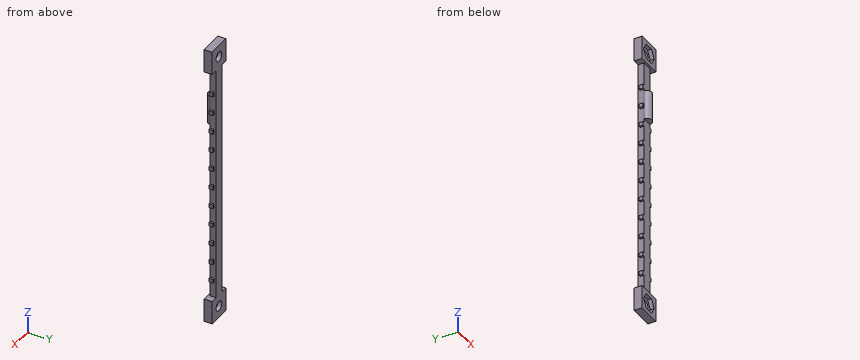
```python
from build123d import *

# Parameters (mm, degrees)
BOSS_EXTRUDE1_DEPTH = 2
BOSS_EXTRUDE2_DEPTH = 1
SKETCH3_W           = 12
SKETCH3_H           = 12
BOSS_EXTRUDE3_DEPTH = 1
CUT_EXTRUDE1_DEPTH  = 2
SKETCH5_R           = 2.5
CUT_EXTRUDE2_DEPTH  = 5
SKETCH6_W           = 3
SKETCH6_H           = 15
BOSS_EXTRUDE4_DEPTH = 5
CUT_EXTRUDE3_DEPTH  = 30
SKETCH9_W           = 3
SKETCH9_H           = 7
CUT_EXTRUDE5_DEPTH  = 20
SKETCH10_W          = 5
SKETCH10_H          = 15
BOSS_EXTRUDE5_DEPTH = 3
CUT_EXTRUDE7_DEPTH  = 20


with BuildPart() as part:
    # Sketch1 → Boss-Extrude1 (new body)
    with BuildSketch(Plane(origin=(0, 0, 0), x_dir=(1, 0, 0), z_dir=(0, 1, 0))):
        Polygon((7.22672382, 6.096), (7.22672382, 18.096), (6.22672382, 18.096), (6.22672382, 20.096), (7.22672382, 20.096), (7.22672382, 28.096), (6.22672382, 28.096), (6.22672382, 30.096), (7.22672382, 30.096), (7.22672382, 38.096), (6.22672382, 38.096), (6.22672382, 40.096), (7.22672382, 40.096), (7.22672382, 48.096), (6.22672382, 48.096), (6.22672382, 50.096), (7.22672382, 50.096), (7.22672382, 58.096), (6.22672382, 58.096), (6.22672382, 60.096), (7.22672382, 60.096), (7.22672382, 68.096), (6.22672382, 68.096), (6.22672382, 70.096), (7.22672382, 70.096), (7.22672382, 78.096), (6.22672382, 78.096), (6.22672382, 80.096), (7.22672382, 80.096), (7.22672382, 88.096), (6.22672382, 88.096), (6.22672382, 90.096), (7.22672382, 90.096), (7.22672382, 98.096), (6.22672382, 98.096), (6.22672382, 100.096), (7.22672382, 100.096), (7.22672382, 108.096), (6.22672382, 108.096), (6.22672382, 110.096), (7.22672382, 110.096), (7.22672382, 118.096), (6.22672382, 118.096), (6.22672382, 120.096), (7.22672382, 120.096), (7.22672382, 128.096), (3.72672382, 128.096), (3.72672382, 140.096), (15.72672382, 140.096), (15.72672382, 128.096), (12.22672382, 128.096), (12.22672382, 120.096), (13.22672382, 120.096), (13.22672382, 118.096), (12.22672382, 118.096), (12.22672382, 110.096), (13.226723821, 110.096), (13.226723821, 108.096), (12.22672382, 108.096), (12.22672382, 100.096), (13.226723821, 100.096), (13.226723821, 98.096), (12.22672382, 98.096), (12.22672382, 90.096), (13.226723821, 90.096), (13.226723821, 88.096), (12.22672382, 88.096), (12.22672382, 80.096), (13.226723821, 80.096), (13.226723821, 78.096), (12.22672382, 78.096), (12.22672382, 70.096), (13.226723821, 70.096), (13.226723821, 68.096), (12.22672382, 68.096), (12.22672382, 60.096), (13.226723821, 60.096), (13.226723821, 58.096), (12.22672382, 58.096), (12.22672382, 50.096), (13.226723821, 50.096), (13.226723821, 48.096), (12.22672382, 48.096), (12.22672382, 40.096), (13.226723821, 40.096), (13.226723821, 38.096), (12.22672382, 38.096), (12.22672382, 30.096), (13.226723821, 30.096), (13.226723821, 28.096), (12.22672382, 28.096), (12.22672382, 20.096), (13.226723821, 20.096), (13.226723821, 18.096), (12.22672382, 18.096), (12.22672382, 6.096), (15.72672382, 6.096), (15.72672382, -5.904), (3.72672382, -5.904), (3.72672382, 6.096), align=None)
    extrude(amount=BOSS_EXTRUDE1_DEPTH)

    # Sketch2 → Boss-Extrude2 (add)
    with BuildSketch(Plane(origin=(0, 2, 0), x_dir=(1, 0, 0), z_dir=(0, 1, 0))):
        Polygon((3.72672382, 140.096), (15.72672382, 140.096), (15.72672382, 128.096), (12.22672382, 128.096), (12.22672382, 6.096), (15.72672382, 6.096), (15.72672382, -5.904), (3.72672382, -5.904), (3.72672382, 6.096), (7.22672382, 6.096), (7.22672382, 128.096), (3.72672382, 128.096), align=None)
    extrude(amount=BOSS_EXTRUDE2_DEPTH)

    # Sketch3 → Boss-Extrude3 (add)
    with BuildSketch(Plane(origin=(0, 0, 0), x_dir=(-1, 0, 0), z_dir=(0, -1, 0))):
        with Locations((-9.72672382, 134.096)):
            Rectangle(SKETCH3_W, SKETCH3_H)
        with Locations((-9.72672382, 0.096)):
            Rectangle(SKETCH3_W, SKETCH3_H)
    extrude(amount=BOSS_EXTRUDE3_DEPTH)

    # Sketch4 → Cut-Extrude1 (cut)
    with BuildSketch(Plane(origin=(0, -1, 0), x_dir=(-1, 0, 0), z_dir=(0, -1, 0))):
        Polygon((-7.365059478, 138.096), (-11.983861632, 138.096), (-14.293262708, 134.096), (-11.983861632, 130.096), (-7.365059478, 130.096), (-5.055658401, 134.096), align=None)
        Polygon((-7.417322744, 4.096), (-12.036124897, 4.096), (-14.345525974, 0.096), (-12.036124897, -3.904), (-7.417322744, -3.904), (-5.107921667, 0.096), align=None)
    extrude(amount=-CUT_EXTRUDE1_DEPTH, mode=Mode.SUBTRACT)

    # Sketch5 → Cut-Extrude2 (cut)
    with BuildSketch(Plane(origin=(0, 1, 0), x_dir=(-1, 0, 0), z_dir=(0, -1, 0))):
        with Locations(Location((-9.72672382, 0.096, 0), (0, 0, 90))):
            Circle(SKETCH5_R)
        with Locations(Location((-9.72672382, 134.096, 0), (0, 0, 90))):
            Circle(SKETCH5_R)
    extrude(amount=-CUT_EXTRUDE2_DEPTH, mode=Mode.SUBTRACT)

    # Sketch6 → Boss-Extrude4 (add)
    with BuildSketch(Plane(origin=(0, 0, 0), x_dir=(-1, 0, 0), z_dir=(0, -1, 0))):
        with Locations((-9.72672382, 28.596)):
            Rectangle(SKETCH6_W, SKETCH6_H)
    extrude(amount=BOSS_EXTRUDE4_DEPTH)

    # Sketch7 → Cut-Extrude3 (cut)
    with BuildSketch(Plane(origin=(0, 0, -36.096), x_dir=(-1, 0, 0), z_dir=(0, 0, -1))):
        with BuildLine():
            Line((-9.72672381, -5), (-8.22672382, -5))
            Line((-8.22672382, -5), (-8.22672382, -1))
            add(Edge.make_bspline(
                [(-9.72672382, -5), (-8.22672382, -5), (-8.22672382, -1)],
                knots=[6.283185307, 6.283185307, 6.283185307, 7.853981634, 7.853981634, 7.853981634], degree=2, weights=[1, 0.707106781, 1]))
        make_face()
        with BuildLine():
            Line((-11.22672382, -5), (-9.72672381, -5))
            add(Edge.make_bspline(
                [(-11.22672382, -1), (-11.22672382, -5), (-9.72672382, -5)],
                knots=[4.71238898, 4.71238898, 4.71238898, 6.283185307, 6.283185307, 6.283185307], degree=2, weights=[1, 0.707106781, 1]))
            Line((-11.22672382, -1), (-11.22672382, -5))
        make_face()
    extrude(amount=-CUT_EXTRUDE3_DEPTH, mode=Mode.SUBTRACT)

    # Sketch9 → Cut-Extrude5 (cut)
    with BuildSketch(Plane.XY.offset(-21.096)):
        with Locations((9.72672382, -3.5)):
            Rectangle(SKETCH9_W, SKETCH9_H)
    extrude(amount=-CUT_EXTRUDE5_DEPTH, mode=Mode.SUBTRACT)

    # Sketch10 → Boss-Extrude5 (add)
    with BuildSketch(Plane(origin=(0, 0, 0), x_dir=(-1, 0, 0), z_dir=(0, -1, 0))):
        with Locations((-9.72672382, 28.596)):
            Rectangle(SKETCH10_W, SKETCH10_H)
    extrude(amount=BOSS_EXTRUDE5_DEPTH)

    # Sketch11 → Cut-Extrude7 (cut)
    with BuildSketch(Plane(origin=(0, 0, -36.096), x_dir=(-1, 0, 0), z_dir=(0, 0, -1))):
        with BuildLine():
            Line((-7.22672382, -3), (-7.22672382, 0))
            ThreePointArc((-7.22672382, 0), (-9.72672382, -2.5), (-12.22672382, 0))
            Line((-12.22672382, 0), (-12.22672382, -3))
            Line((-12.22672382, -3), (-7.22672382, -3))
        make_face()
    extrude(amount=-CUT_EXTRUDE7_DEPTH, mode=Mode.SUBTRACT)


solid = part.part
```
Part model, mm, in its own coordinate system. Coordinates: 2 decimals unless noted, no trailing zeros. Loops run counter-clockwise (first coordinate to the right, second up) from the corner with the lowest first, then second, coordinate; pieces in that order, holes last. Notation, with made-up numbers: (1.25, -13.5) - (50.25, -13.5) arc R21 ccw to (50.25, -6.5) - close; hole circle Ø3 at (-12, 34.25). An arc over 180 degrees is marked (long way). Write item = value, one per line. Start each with the question number.
Item 1: Wall check: L1, parallel to Z at x = 11.5, y = 0.8; L2, parallel to Z at x = 10, y = 2.45; L3, parallel to X at y = 2.55, z = -73. Give the ranges that are in metal, low to high. Write a range as from..to.
Item 2: Cut at A-A, the plane z = -53. Give the cut face in (x, y), and give its area (3 significant figures).
Item 3: Flat gauge pins, fed straight in: pin 1 Ø3 at (y, z) = (1, -31.5) entering from -X; pin 2 Ø1.5 at (y, z) = (2, -96) entering from +X; pin 3 Ø0.8 at (x, z) = (13, -79) entering from +Y. Where does each tip first touch, or does it go through?
The answers:
q1.L1 = -140.1..-138.1, -130.1..-4.1, 3.9..5.9
q1.L2 = -140.1..-136.58, -131.61..-2.58, 2.39..5.9
q1.L3 = 7.23..12.23
q2.outline = (7.23, 0) - (12.23, 0) - (12.23, 3) - (7.23, 3) - close
q2.area = 15.0 mm2
q3.pin_1 = 6.23
q3.pin_2 = 12.23
q3.pin_3 = 2
